from build123d import *

# Parameters (mm, degrees)
CYLINDER005_R          = 2.25
CYLINDER005_DEPTH      = 3
CYLINDER005_ROLL_ANGLE = 90
CYLINDER006_R          = 2.25
CYLINDER006_DEPTH      = 3
CYLINDER006_ROLL_ANGLE = 90
CYLINDER004_R          = 2.25
CYLINDER004_DEPTH      = 3
CYLINDER004_ROLL_ANGLE = 90
BOX011_W               = 15
BOX011_H               = 3
BOX011_DEPTH           = 60
BOX010_W               = 3
BOX010_H               = 3
BOX010_DEPTH           = 3
BOX009_W               = 9
BOX009_H               = 3
BOX009_DEPTH           = 9
BOX013_W               = 3
BOX013_H               = 3
BOX013_DEPTH           = 3
BOX012_W               = 9
BOX012_H               = 3
BOX012_DEPTH           = 9


with BuildPart() as cylinder005:
    # Cylinder005 → Cylinder005 (new body)
    with BuildSketch(Plane.XY):
        Circle(CYLINDER005_R)
    extrude(amount=CYLINDER005_DEPTH)


with BuildPart() as cylinder005_1:
    # Cylinder005 roll: moved
    add(cylinder005.part.rotate(Axis((0, 0, 0), (1, 0, 0)), CYLINDER005_ROLL_ANGLE))


with BuildPart() as cylinder005_2:
    # Cylinder005 placement: moved
    add(cylinder005_1.part.moved(Location((0, -63, -3))))


with BuildPart() as cylinder006:
    # Cylinder006 → Cylinder006 (new body)
    with BuildSketch(Plane.XY):
        Circle(CYLINDER006_R)
    extrude(amount=CYLINDER006_DEPTH)


with BuildPart() as cylinder006_1:
    # Cylinder006 roll: moved
    add(cylinder006.part.rotate(Axis((0, 0, 0), (1, 0, 0)), CYLINDER006_ROLL_ANGLE))


with BuildPart() as cylinder006_2:
    # Cylinder006 placement: moved
    add(cylinder006_1.part.moved(Location((0, -63, -21))))


with BuildPart() as cylinder004:
    # Cylinder004 → Cylinder004 (new body)
    with BuildSketch(Plane.XY):
        Circle(CYLINDER004_R)
    extrude(amount=CYLINDER004_DEPTH)


with BuildPart() as cylinder004_1:
    # Cylinder004 roll: moved
    add(cylinder004.part.rotate(Axis((0, 0, 0), (1, 0, 0)), CYLINDER004_ROLL_ANGLE))


with BuildPart() as cylinder004_2:
    # Cylinder004 placement: moved
    add(cylinder004_1.part.moved(Location((0, -63, -12))))


with BuildPart() as cube011:
    # Box011 → Box011 (new body)
    with BuildSketch(Plane(origin=(-7.5, -66, -27), x_dir=(1, 0, 0), z_dir=(0, 0, 1))):
        with Locations((7.5, 1.5)):
            Rectangle(BOX011_W, BOX011_H)
    extrude(amount=BOX011_DEPTH)


with BuildPart() as cube010:
    # Box010 → Box010 (new body)
    with BuildSketch(Plane(origin=(-1.5, -66, 6), x_dir=(1, 0, 0), z_dir=(0, 0, 1))):
        with Locations((1.5, 1.5)):
            Rectangle(BOX010_W, BOX010_H)
    extrude(amount=BOX010_DEPTH)


with BuildPart() as cut010:
    # Box009 → Box009 (new body)
    with BuildSketch(Plane(origin=(-4.5, -66, 3), x_dir=(1, 0, 0), z_dir=(0, 0, 1))):
        with Locations((4.5, 1.5)):
            Rectangle(BOX009_W, BOX009_H)
    extrude(amount=BOX009_DEPTH)

    # Cut010: cut Cube010
    add(cube010.part, mode=Mode.SUBTRACT)


with BuildPart() as cut010_1:
    # Cut010 placement: moved
    add(cut010.part.moved(Location((0, 0, 30))))


with BuildPart() as cube013:
    # Box013 → Box013 (new body)
    with BuildSketch(Plane(origin=(-1.5, -66, 6), x_dir=(1, 0, 0), z_dir=(0, 0, 1))):
        with Locations((1.5, 1.5)):
            Rectangle(BOX013_W, BOX013_H)
    extrude(amount=BOX013_DEPTH)


with BuildPart() as pitchringconnector:
    # Box012 → Box012 (new body)
    with BuildSketch(Plane(origin=(-4.5, -66, 3), x_dir=(1, 0, 0), z_dir=(0, 0, 1))):
        with Locations((4.5, 1.5)):
            Rectangle(BOX012_W, BOX012_H)
    extrude(amount=BOX012_DEPTH)

    # Cut011: cut Cube013
    add(cube013.part, mode=Mode.SUBTRACT)


with BuildPart() as pitchringconnector_1:
    # Cut011 placement: moved
    add(pitchringconnector.part.moved(Location((0, 0, -39))))

    # Fusion: union Cube011, Cut010
    add(cube011.part)
    add(cut010_1.part)

    # Cut012: cut Cylinder004
    add(cylinder004_2.part, mode=Mode.SUBTRACT)

    # Cut013: cut Cylinder006
    add(cylinder006_2.part, mode=Mode.SUBTRACT)

    # Cut014: cut Cylinder005
    add(cylinder005_2.part, mode=Mode.SUBTRACT)


with BuildPart() as pitchringconnector_2:
    # Cut014 placement: moved
    add(pitchringconnector_1.part.moved(Location((0, 29, -3))))


solid = pitchringconnector_2.part
Model file for the job. Use its own axes, mm. A direction names the side the tool comes from. Coordinates: 2 decimals unless noted, no trailing zeros. Write each loop counter-clockwise with the first axis right and the second up, starting at its lowest first coordinate (ties: lowest second). Pieces come first, ordered by that corner, then holes. Notation, with made-up numbers: (30.5, 38) -> (40.5, 38) arc R26 ccw to (40.5, 62) -> close; hole circle Ø1 at (7, 8.25). An arc over 180 degrees is marked (long way). One line per item, written item: value. Start each with the question number.
1) Flat gauge pins, fed straight in: pin 1 Ø0.9 at (y, z) = (-35.5, -35) entering from +X; pin 2 Ø0.9 at (x, y) = (-6.5, -36) entering from +Z; pin 3 Ø0.9 at (y, z) = (-36, -34) entering from -X. Where does each tip first touch, or does it go through?
2) Slice it at D-D on x = 6.75. Write the cut outline in (y, z).
3) Slice it at C-C on y = -34.7. Write the cut outline in (x, z), then the cut area to 3 significant figures.
4) Slice it at A-A on x = 0. Write the cut outline in (y, z), then the cut area to 4 significant figures.
5) Pull direction X, two halves, no side cores. Call faces 4 (the face through (-4.5, -36, 34)), 5 (the face through (0, -35, -39)), 6 (the face through (-1.5, -36, 34)): +X half, -X half, draft (parallel to the pull), parting line (faces both ways), or undercut.
6) Which spindle directions (+Z, -Z, +X, -X, +Y, -Y) get a long thin tool onto all of the face, cutting with end or side? Do faces 1 (the face through (-6, -35, -30)), 2 (the face through (6, -35, -30)), 3 (the face through (0, -35, -36)). Say none if no direction does.
7) Slice it at B-B on z = -24. Write the cut outline in (x, y), then the cut area to 3 significant figures.
8) Probe probe 1 along Z at (x, y) = (0, -34.85); probe 2 along Z at (x, y) = (1.25, -36.6); probe 3 along Z at (x, y) = (-5.5, -34.85). List the from-to ranges inside material, lowest first.
Answers follow:
1. pin 1: x = 4.5
1. pin 2: z = 30
1. pin 3: x = -4.5
2. outline: (-37, -30) -> (-34, -30) -> (-34, 30) -> (-37, 30) -> close
3. outline: (-7.5, -30) -> (-4.5, -30) -> (-4.5, -39) -> (4.5, -39) -> (4.5, -30) -> (7.5, -30) -> (7.5, 30) -> (4.5, 30) -> (4.5, 39) -> (-4.5, 39) -> (-4.5, 30) -> (-7.5, 30) -> close; hole circle Ø4.5 at (0, -24); hole circle Ø4.5 at (0, -15); hole circle Ø4.5 at (0, -6); hole (-1.5, -36) -> (1.5, -36) -> (1.5, -33) -> (-1.5, -33) -> close; hole (-1.5, 33) -> (1.5, 33) -> (1.5, 36) -> (-1.5, 36) -> close
3. area: 996 mm2
4. outline: (-37, -39) -> (-34, -39) -> (-34, -36) -> (-37, -36) -> close; (-37, -33) -> (-34, -33) -> (-34, -26.25) -> (-37, -26.25) -> close; (-37, -21.75) -> (-34, -21.75) -> (-34, -17.25) -> (-37, -17.25) -> close; (-37, -12.75) -> (-34, -12.75) -> (-34, -8.25) -> (-37, -8.25) -> close; (-37, -3.75) -> (-34, -3.75) -> (-34, 33) -> (-37, 33) -> close; (-37, 36) -> (-34, 36) -> (-34, 39) -> (-37, 39) -> close
4. area: 175.5 mm2
5. face 4: -X half
5. face 5: draft
5. face 6: undercut
6. face 1: -Z, -X, +Y, -Y
6. face 2: -Z, +X, +Y, -Y
6. face 3: +Y, -Y
7. outline: (-7.5, -37) -> (-2.25, -37) -> (-2.25, -34) -> (-7.5, -34) -> close; (2.25, -37) -> (7.5, -37) -> (7.5, -34) -> (2.25, -34) -> close
7. area: 31.5 mm2
8. probe 1: -39 to -36, -33 to -26.25, -21.75 to -17.25, -12.75 to -8.25, -3.75 to 33, 36 to 39
8. probe 2: -39 to -36, -33 to -25.87, -22.13 to -16.87, -13.13 to -7.87, -4.13 to 33, 36 to 39
8. probe 3: -30 to 30
